Print and shaded views of the part. All mm, measured from the part's lowest x, y and z. A direction names the side the tool comes from. Round coordinates to 2 decimals unless told otherwise and drop trailing zeros. Write each loop counter-clockwise with the first axis right and the second up, starting at its lowest first coordinate (ties: lowest second). Pieces come first, ordered by that corner, then holes. Notation, with made-up numbers: (77, 4.5) - (109, 4.5) arc R31 cw to (109, 39.5) - close; hole circle Ø5 at (25.5, -6.75). An arc over 180 degrees is marked (long way). One line per item, written item: value.
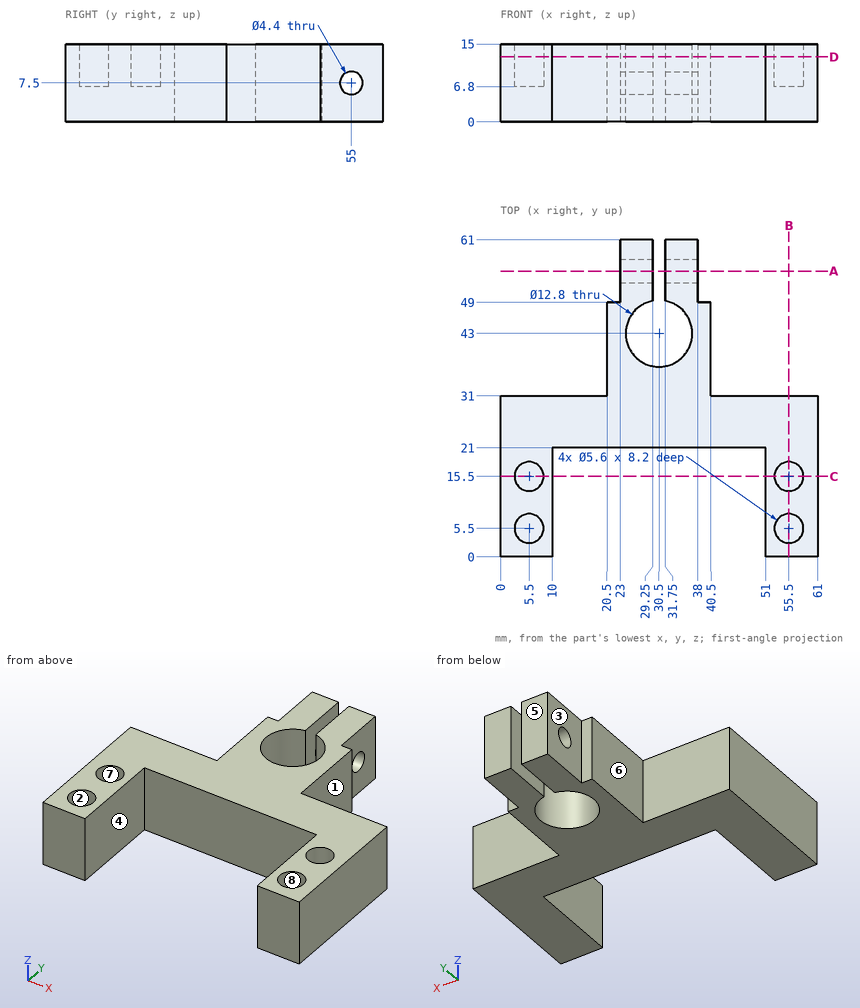
1. Tool access for the marked faces 1, 2, 3 and 4: list every direction of +Z, -Z, +X, -X, +Y, -Y with a clear straight run to the whole face (end or side of a thin tool).
Report:
face 1: +Z, -Z, +X, +Y
face 2: +Z
face 3: +Z, -Z, -X, +Y
face 4: +Z, -Z, -Y
2. Band-saw the part on D-D on z = 12.5. Write the cut outline in (x, y).
Report:
outline: (0, 0) - (10, 0) - (10, 21) - (51, 21) - (51, 0) - (61, 0) - (61, 31) - (40.5, 31) - (40.5, 49) - (38, 49) - (38, 61) - (31.75, 61) - (31.75, 49.28) arc R6.4 cw (long way) to (29.25, 49.28) - (29.25, 61) - (23, 61) - (23, 49) - (20.5, 49) - (20.5, 31) - (0, 31) - close; hole circle Ø5.6 at (5.5, 5.5); hole circle Ø5.6 at (5.5, 15.5); hole circle Ø5.6 at (55.5, 5.5); hole circle Ø5.6 at (55.5, 15.5)
3. Drop flat-ended pins along their axis: pin 1 (3 mm diameter, centred on x = 55.5, y = 7, fed in from +Z); pin 2 (5 mm diameter, centred on y = 36, z = 5, fed in from -X); pin 3 (7.5 mm diameter, centred on y = 44.5, z = 8, fed in from +X); pin 4 (1.2 mm diameter, centred on x = 39, z = 5.5, fed in from +Y). Give the stop position or say it passes through.
Report:
pin 1: z = 15
pin 2: x = 20.5
pin 3: x = 40.5
pin 4: y = 49
4. Band-saw the part on C-C on y = 15.5. Write the cut outline in (x, z).
Report:
outline: (0, 0) - (10, 0) - (10, 15) - (8.3, 15) - (8.3, 6.8) - (2.7, 6.8) - (2.7, 15) - (0, 15) - close; (51, 0) - (61, 0) - (61, 15) - (58.3, 15) - (58.3, 6.8) - (52.7, 6.8) - (52.7, 15) - (51, 15) - close
5. Band-saw the part on B-B on x = 55.5. Write the cut outline in (y, z).
Report:
outline: (0, 0) - (31, 0) - (31, 15) - (18.3, 15) - (18.3, 6.8) - (12.7, 6.8) - (12.7, 15) - (8.3, 15) - (8.3, 6.8) - (2.7, 6.8) - (2.7, 15) - (0, 15) - close
6. Band-saw the part on A-A on y = 55. Write the cut outline in (x, z), plus the area to 4 significant figures.
Report:
outline: (23, 0) - (29.25, 0) - (29.25, 5.3) - (23, 5.3) - close; (23, 9.7) - (29.25, 9.7) - (29.25, 15) - (23, 15) - close; (31.75, 0) - (38, 0) - (38, 5.3) - (31.75, 5.3) - close; (31.75, 9.7) - (38, 9.7) - (38, 15) - (31.75, 15) - close
area: 132.5 mm²
7. Wall check: probe 1 along Y at (x, z) = (55.5, 11.25); probe 2 along X at (y, z) = (50.5, 2); probe 3 along X at (y, z) = (13, 14.25). Give the ranges that are in metal, low to high. Write a range as [from, to].
Report:
probe 1: [0, 2.7], [8.3, 12.7], [18.3, 31]
probe 2: [23, 29.25], [31.75, 38]
probe 3: [0, 4.24], [6.76, 10], [51, 54.24], [56.76, 61]
8. Mould opens along Y. For the marked faces 5, 6, 7 and 8 say: released by +Y, released by -Y, zero draft, split by the parting line, or undercut.
Report:
face 5: released by +Y
face 6: zero draft
face 7: undercut
face 8: undercut
